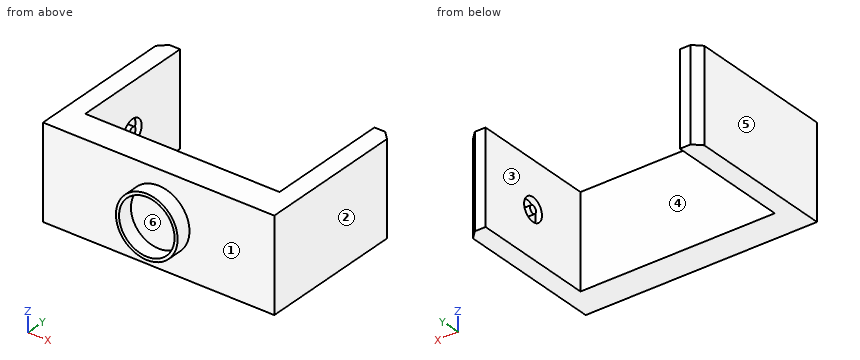
from build123d import *

# Parameters (mm, degrees)
EXTRUDE_1_DEPTH     = 30
SKETCH_2_R          = 20
SKETCH_2_R_2        = 18
EXTRUDE_2_DEPTH     = 10
SKETCH_3_R          = 7.5
SKETCH_3_R_2        = 2.5
CUT_EXTRUDE_1_DEPTH = 4


with BuildPart() as part:
    # 草图1 → 凸台-拉伸1 (new, symmetric)
    with BuildSketch(Plane.XY):
        Polygon((-63, 100), (-70, 100), (-75, 95), (-75, 0), (0, 0), (0, 20), (-63, 20), align=None)
        Polygon((63, 20), (0, 20), (0, 0), (75, 0), (75, 95), (70, 100), (63, 100), align=None)
    extrude(amount=EXTRUDE_1_DEPTH, both=True)

    # 草图2 → 凸台-拉伸2 (add)
    with BuildSketch(Plane.XZ):
        with Locations(Location((0, 0, 0), (0, 0, 180))):
            Circle(SKETCH_2_R)
        Circle(SKETCH_2_R_2, mode=Mode.SUBTRACT)
    extrude(amount=EXTRUDE_2_DEPTH)

    # 草图3 → 切除-拉伸1 (cut)
    with BuildSketch(Plane(origin=(-63, 0, 0), x_dir=(0, 0, -1), z_dir=(1, 0, 0))):
        with Locations(Location((0, 60, 0), (0, 0, 90))):
            Circle(SKETCH_3_R)
        with Locations(Location((0, 60, 0), (0, 0, 90))):
            Circle(SKETCH_3_R_2, mode=Mode.SUBTRACT)
    cut_extrude_1 = extrude(amount=-CUT_EXTRUDE_1_DEPTH, mode=Mode.SUBTRACT)

    # 镜向1: 切除-拉伸1 across plane
    add(cut_extrude_1.mirror(Plane(origin=(0, 0, 0), x_dir=(0, 0, 1), z_dir=(1, 0, 0))), mode=Mode.SUBTRACT)


solid = part.part
Can you work these out from the model? Positions are in its coordinate system, mm. Face numbers are marked on the shaded views. A direction names the side the tool comes from. Round coordinates to 2 decimals unless told otherwise and drop trailing zeros. Write each loop counter-clockwise with the first axis right and the second up, starting at its lowest first coordinate (ties: lowest second). Pieces come first, ordered by that corner, then holes. Notation, with made-up numbers: (24, -14) -> (58, -14) arc R25 ccw to (58, 3) -> close; hole circle Ø1 at (8, 88.25). An arc over 180 degrees is marked (long way). One line per question, with ' | ' between items. Start each with the question number.
1) Suppose I cut it at A-A on y = 60. Write out the boundary of the cut face in (x, z).
2) On a 3-axis mill with a long thin cutter (end or side, diameter ignored), from which of +Z, -Z, +X, -X, +Y, -Y can I reach the whole of each face in a straight line? I mean the marked faces 4, 5 and 6. Say none if no direction works.
3) If we mould it in two halves opening along X, with no side actions, what happens to the marked faces 1, 2 and 3? For each: released by +X, released by -X, zero draft, split by the parting line, or undercut.
4) Suppose I cut it at D-D on y = 73. Write out the boundary of the cut face in (x, z).
5) I'm going to push flat-ended pins straight in: P1, Ø10, axis at x = -25.5, z = 5.5, coming from the +Y side; P2, Ø18, axis at x = -1, z = -6.5, coming from the -Y side. Where does each tip first touch, or does it pass through?
6) Suppose I cut it at C-C on x = 0. Write out the boundary of the cut face in (y, z), then the cut area to 3 significant figures.
7) I need wall thicknesses on line 1 (Z direction, x = 66.1, y = 60); line 2 (X direction, y = 25, z = 25); line 3 (Z direction, x = 0, y = -2.25). Which ranges of each line are inside material? Lowest first, please. Write a range as [from, to].
Return value:
1) outline: (-75, -30) -> (-63, -30) -> (-63, -7.5) -> (-67, -7.5) -> (-67, -2.5) -> (-63, -2.5) -> (-63, 2.5) -> (-67, 2.5) -> (-67, 7.5) -> (-63, 7.5) -> (-63, 30) -> (-75, 30) -> close; (63, -30) -> (75, -30) -> (75, 30) -> (63, 30) -> (63, 7.5) -> (67, 7.5) -> (67, 2.5) -> (63, 2.5) -> (63, -2.5) -> (67, -2.5) -> (67, -7.5) -> (63, -7.5) -> close
2) face 4: +Z, -Z, +Y | face 5: +Z, -Z, -X, +Y, -Y | face 6: -Y
3) face 1: zero draft | face 2: released by +X | face 3: undercut
4) outline: (-75, -30) -> (-63, -30) -> (-63, 30) -> (-75, 30) -> close; (63, -30) -> (75, -30) -> (75, 30) -> (63, 30) -> close
5) P1: stops at y = 20 | P2: stops at y = 0
6) outline: (-10, -20) -> (0, -20) -> (0, -30) -> (20, -30) -> (20, 30) -> (0, 30) -> (0, 20) -> (-10, 20) -> (-10, 18) -> (0, 18) -> (0, -18) -> (-10, -18) -> close | area: 1,240 mm2
7) line 1: z = [-30, -7.5], [-2.5, 2.5], [7.5, 30] | line 2: x = [-75, -63], [63, 75] | line 3: z = [-20, -18], [18, 20]
